For this review, take the finished solid that the model builds, in its own axes (mm). Face numbers are marked on the shaded views. A direction names the side the tool comes from. Round coordinates to 2 decimals unless told otherwise and drop trailing zeros. Order: outer loops, then holes, each group sorted by start corner. A loop starts at its lowest first (then second) coordinate and runs counter-clockwise, first axis right, second up. Notation, with made-up numbers: (-2.5, -37.5) - (27.5, -37.5) arc R26 cw to (27.5, -21.5) - close; hole circle Ø11 at (-31.75, 17.5). An arc over 180 degrees is marked (long way). Write each question's results on one line, items separated by ' | '. Start each with the question number.
(1) Insertion check: pin 1 Ø5 at (x, z) = (-4, -151) entering from +Y; pin 2 Ø8.5 at (x, y) = (-48, 4.5) entering from +Z. Each pin has a flat end and moves straight along its axis. Give the tip position at first contact, or say it passes through.
(2) Take a section at C-C, the plane z = -140. Give the boundary of the cut face in (x, y).
(3) For L1, parallel to X at y = -0.85, z = -151; L2, parallel to Z at x = -4, y = -0.65; L3, parallel to Y at x = -33, z = -32, list the stretches that pass through material, from the lowest coordinate up. Write a range as from..to.
(4) Take a section at A-A, the plane x = -72. Give the boundary of the cut face in (y, z), plus the area to 3 significant figures.
(5) For the marked faces 1, 2 and 3, list the 3-axis set-ups (+Z, -Z, +X, -X, +Y, -Y) from which the entire face can be reached by the end or side of a thin tool; tool diameter is ignored.
(6) Take a section at B-B, the plane z = -4. Give the boundary of the cut face in (x, y).
(7) Take a section at D-D, the plane y = 2.5. Give the boundary of the cut face in (x, z), plus the area to 4 significant figures.
Autodesk Inventor part; units mm, degrees
ref_plane "YZ Plane" through (0, 0, 0) normal (1, 0, 0) x (0, 1, 0)
ref_plane "XZ Plane" through (0, 0, 0) normal (0, 1, 0) x (-1, 0, 0)
ref_plane "XY Plane" through (0, 0, 0) normal (0, 0, 1) x (1, 0, 0)
sketch "Sketch1" plane through (0, 0, 0) normal (0, 1, 0) x (-1, 0, 0)
  line L0 (0, 0) -> (76, 0)
  line L1 (76, 0) -> (76, -155)
  line L2 (76, -155) -> (0, -155)
  line L3 (0, -155) -> (0, 0)
  line L4 (81.1574, -77.5) -> (-13.3813, -77.5) construction
  line L5 (38, 8.4809) -> (38, -161.1275) construction
  line L6 (4, -151) -> (72, -151) construction
  line L7 (72, -151) -> (72, -4) construction
  line L8 (72, -4) -> (4, -4) construction
  line L9 (4, -4) -> (4, -151) construction
  line L10 (4, -151) -> (72, -4) construction
  line L11 (72, -151) -> (4, -4) construction
  circle A0 centre (72, -4) radius 1.55
  circle A1 centre (72, -151) radius 1.55
  circle A2 centre (4, -151) radius 1.55
  circle A3 centre (4, -4) radius 1.55
  point P0 (76, -77.5)
  point P1 (38, -155)
  point P2 (38, -77.5)
  dimension "d0" = 76
  dimension "d1" = 155
  dimension "d2" = 68
  dimension "d3" = 147
  dimension "d4" = 3.1
  dimension "d5" = 3.1
  dimension "d6" = 3.1
  dimension "d7" = 3.1
extrude "Extrusion1" add sketch "Sketch1" against normal blind 1.65
sketch "Sketch2" plane through (0, 0, 0) normal (0, 1, 0) x (1, 0, 0)
  line L0 (-61, 99) -> (-36, 99)
  line L1 (-36, 99) -> (-36, 154)
  line L2 (-36, 154) -> (-61, 154)
  line L3 (-61, 154) -> (-61, 99)
  line L4 (0, 155) -> (-76, 155)
  line L5 (-76, 155) -> (-76, 0)
  point P0 (0, 0)
  dimension "d10" = 25
  dimension "d11" = 55
  dimension "d12" = 56
  dimension "d13" = 40
extrude "Extrusion2" add sketch "Sketch2" along normal blind 17
properties part number "Coms Board V1"
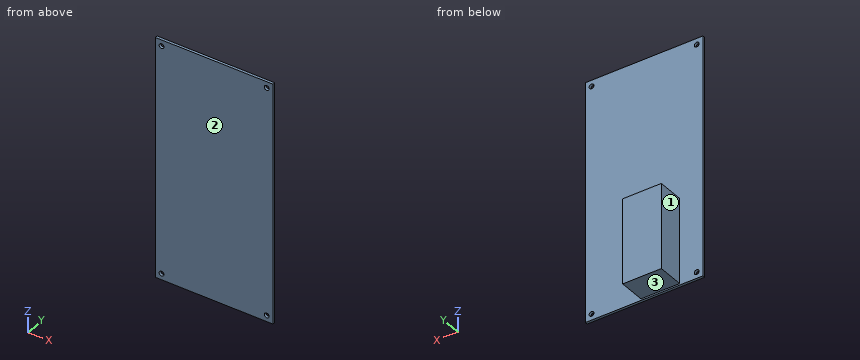
Results below:
1) pin 1: stops at y = 0 | pin 2: stops at z = -99
2) outline: (-76, -1.65) - (0, -1.65) - (0, 0) - (-36, 0) - (-36, 17) - (-61, 17) - (-61, 0) - (-76, 0) - close
3) L1: x = -76..-73.55, -70.45..-5.55, -2.45..0 | L2: z = -155..-152.55, -149.45..-5.55, -2.45..0 | L3: y = -1.65..0
4) outline: (-1.65, -155) - (0, -155) - (0, -152.55) - (-1.65, -152.55) - close; (-1.65, -149.45) - (0, -149.45) - (0, -5.55) - (-1.65, -5.55) - close; (-1.65, -2.45) - (0, -2.45) - (0, 0) - (-1.65, 0) - close | area: 246 mm^2
5) face 1: +Z, -Z, -X, +Y | face 2: +Z, -Z, +X, -X, -Y | face 3: -Z, +X, -X, +Y
6) outline: (-76, -1.65) - (-73.55, -1.65) - (-73.55, 0) - (-76, 0) - close; (-70.45, -1.65) - (-5.55, -1.65) - (-5.55, 0) - (-70.45, 0) - close; (-2.45, -1.65) - (0, -1.65) - (0, 0) - (-2.45, 0) - close
7) outline: (-61, -154) - (-36, -154) - (-36, -99) - (-61, -99) - close | area: 1,375 mm^2
